Verification items for the finished model (mm, model axes). A direction names the side the tool comes from. Give positions to 0.01 mm unless a question says otherwise; leave off trailing zeros. Write each loop counter-clockwise with the first axis right and the second up, starting at its lowest first coordinate (ties: lowest second). Pieces come first, ordered by that corner, then holes. Notation, with made-up numbers: (4, 19) - (40, 19) arc R9 ccw to (40, 27) - close; hole circle Ø4 at (74, -27.5). An arc over 180 degrees is marked (long way). Answer as a JSON object with one key per item and string values. Group by question number.
Item 1: Go/stop test with flat-tipped pins: pin 1 (3 mm diameter, centred on y = 7, z = 29, fed in from -X); pin 2 (8 mm diameter, centred on x = -18, y = -17, fed in from +Z); pin 3 (12 mm diameter, centred on x = 20.5, z = 31.5, fed in from -Y); pin 4 (10 mm diameter, centred on y = -16, z = 11.5, fed in from -X). Record where each tip stops, or that it passes through.
Item 2: Sectioned sample at A-A, the plane y = -16. Record the boundary of the cut face in (x, z), and give its area (3 significant figures).
Item 3: Sectioned sample at B-B, the plane z = 0. Record the boundary of the cut face in (x, y).
Item 4: Scan lines: line 1 along Z through (x, y) = (-12.5, -17.5); line 2 along X through (y, z) = (-9, 1); line 3 along Y through (x, z) = (2.5, 11). Record each from-to range of solid material in increasing order. Write a range as [from, to].
Item 5: Sectioned sample at C-C, the plane x = 51. Record the boundary of the cut face in (y, z), and give its area (3 significant figures).
Item 6: Tool access check on faces 1 (the face through (56, 0, 32.5)), 2 (the face through (-2, -6.25, 23)), 3 (the face through (37, -25, 32)), 4 (the face through (37, 25, 32)), 5 (the face through (25.77, 15.49, 39.66)). Record the directions out of +Z, -Z, +X, -X, +Y, -Y that give a thin tool (end or side, any length) a straight path to the whole face; none if there is none.
```python
from build123d import *

# Parameters (mm, degrees)
F1_DEPTH = 62.5
F0_W     = 20
F0_H     = 15
F2_DEPTH = 25
F3_DEPTH = 6.25


with BuildPart() as f1:
    # F0 (on Front) → F1 (new body, symmetric)
    with BuildSketch(Plane.XZ):
        Polygon((17.5, 7.5), (-32.5, 7.5), (-32.5, -7.5), (32.5, -7.5), (32.5, 7.5), align=None)
    extrude(amount=F1_DEPTH, both=True)

    # F0 (on Front) → F2 (join, symmetric)
    with BuildSketch(Plane.XZ):
        with BuildLine():
            Line((17.5, 20), (17.5, 7.5))
            Line((17.5, 7.5), (32.5, 7.5))
            Line((32.5, 7.5), (32.5, 20))
            ThreePointArc((32.5, 20), (36.1611652352, 28.8388347648), (45, 32.5))
            Line((45, 32.5), (47.5, 32.5))
            Line((47.5, 32.5), (47.5, 47.5))
            Line((47.5, 47.5), (45, 47.5))
            ThreePointArc((45, 47.5), (25.5545635174, 39.4454364826), (17.5, 20))
        make_face()
        with Locations((57.5, 40)):
            Rectangle(F0_W, F0_H)
    extrude(amount=F2_DEPTH, both=True)

    # F0 (on Front) → F3 (join, symmetric)
    with BuildSketch(Plane.XZ):
        with BuildLine():
            add(Edge.make_bspline(
                [(-32.5, 7.5), (-32.5, 26.5529304743), (7.5689763762, 47.5), (45, 47.5)],
                knots=[0, 0, 0, 0, 87.2138177126, 87.2138177126, 87.2138177126, 87.2138177126], degree=3))
            Line((-32.5, 7.5), (17.5, 7.5))
            Line((17.5, 7.5), (17.5, 20))
            ThreePointArc((17.5, 20), (25.5545635174, 39.4454364826), (45, 47.5))
        make_face()
    extrude(amount=F3_DEPTH, both=True)


solid = f1.part
```
Geometry check:
{
 "1": {"pin 1": "x = -18.98", "pin 2": "z = 7.5", "pin 3": "y = -25", "pin 4": "x = -32.5"},
 "2": {"outline": "(-32.5, -7.5) - (32.5, -7.5) - (32.5, 20) arc R12.5 cw to (45, 32.5) - (67.5, 32.5) - (67.5, 47.5) - (45, 47.5) arc R27.5 ccw to (17.5, 20) - (17.5, 7.5) - (-32.5, 7.5) - close", "area": "1,970 mm^2"},
 "3": {"outline": "(-32.5, -62.5) - (32.5, -62.5) - (32.5, 62.5) - (-32.5, 62.5) - close"},
 "4": {"line 1": "[-7.5, 7.5]", "line 2": "[-32.5, 32.5]", "line 3": "[-6.25, 6.25]"},
 "5": {"outline": "(-25, 32.5) - (25, 32.5) - (25, 47.5) - (-25, 47.5) - close", "area": "750 mm^2"},
 "6": {"face 1": "-Z, +X, +Y, -Y", "face 2": "+Z, -X, -Y", "face 3": "+Z, +X, -X, -Y", "face 4": "+Z, +X, -X, +Y", "face 5": "+Z, -X, +Y"}
}
